Can you work these out from the model? Positions are in its coordinate system, mm. Round coordinates to 2 decimals unless told otherwise and drop trailing zeros. Loops run counter-clockwise (first coordinate to the right, second up) from the corner with the lowest first, then second, coordinate; pieces in that order, holes last.
(1) Thinking about a two-plate mould opening in Z: for faces 1 (the face through (0, 1, 30)), 2 (the face through (15.364, 0.72, -15.975)), 3 (the face through (1.936, 0.72, -13.536)), 4 (the face through (30, 1, 0)), which applies, released by +Z, released by -Z, zero draft, split by the parting line, or undercut?
(2) If I drill on line 1 along X through (y, z) = (0.4, 0) (3 decimals); line 2 along Z through (x, y) = (-14.96, 1.2) (3 decimals); line 3 along Z through (x, y) = (-27, 0.4), over which ranges is the centre line in solid material (lowest first)?
(3) I want a section at C-C on y = 0.5. Give the number of separate pieces and of enclosed holes in the cut face, plus the area to 3 significant figures.
(4) I want a section at B-B on z = 0. Write out the boundary of the cut face in (x, y) (3 decimals), plus the area to 3 significant figures.
(5) I want a section at A-A on z = 15. Write out the boundary of the cut face in (x, y) (3 decimals).
from build123d import *

# Parameters (mm, degrees)
SKETCH1_W           = 60
SKETCH1_H           = 60
SKETCH1_R           = 0.55
SKETCH1_R_2         = 1.465
SKETCH1_R_3         = 1.375
SKETCH1_R_4         = 1.055
BOSS_EXTRUDE1_DEPTH = 1.46


with BuildPart() as part:
    # Sketch1 → Boss-Extrude1 (new body)
    with BuildSketch(Plane(origin=(0, 0, 0), x_dir=(1, 0, 0), z_dir=(0, 1, 0))):
        Rectangle(SKETCH1_W, SKETCH1_H)
        with Locations(Location((-28.5, 28.5, 0), (0, 0, 270))):
            Circle(SKETCH1_R, mode=Mode.SUBTRACT)
        with Locations(Location((-27.968, 15, 0), (0, 0, 270))):
            Circle(SKETCH1_R_2, mode=Mode.SUBTRACT)
        with Locations(Location((-14.75, 0, 0), (0, 0, 270))):
            Circle(SKETCH1_R_3, mode=Mode.SUBTRACT)
        with Locations(Location((-14.960000108, 15, 0), (0, 0, 270))):
            Circle(SKETCH1_R_4, mode=Mode.SUBTRACT)
        with Locations(Location((-2, 15, 0), (0, 0, 270))):
            Circle(SKETCH1_R_2, mode=Mode.SUBTRACT)
        with Locations(Location((2, 15, 0), (0, 0, 90))):
            Circle(SKETCH1_R_2, mode=Mode.SUBTRACT)
        with Locations(Location((14.960000108, 15, 0), (0, 0, 90))):
            Circle(SKETCH1_R_4, mode=Mode.SUBTRACT)
        with Locations(Location((14.75, 0, 0), (0, 0, 90))):
            Circle(SKETCH1_R_3, mode=Mode.SUBTRACT)
        with Locations(Location((27.968, 15, 0), (0, 0, 90))):
            Circle(SKETCH1_R_2, mode=Mode.SUBTRACT)
        with Locations(Location((28.5, 28.5, 0), (0, 0, 90))):
            Circle(SKETCH1_R, mode=Mode.SUBTRACT)
        with Locations(Location((28.5, -28.5, 0), (0, 0, 270))):
            Circle(SKETCH1_R, mode=Mode.SUBTRACT)
        with Locations(Location((27.968, -15, 0), (0, 0, 270))):
            Circle(SKETCH1_R_2, mode=Mode.SUBTRACT)
        with Locations(Location((14.960000108, -15, 0), (0, 0, 270))):
            Circle(SKETCH1_R_4, mode=Mode.SUBTRACT)
        with Locations(Location((2, -15, 0), (0, 0, 270))):
            Circle(SKETCH1_R_2, mode=Mode.SUBTRACT)
        with Locations(Location((-2, -15, 0), (0, 0, 90))):
            Circle(SKETCH1_R_2, mode=Mode.SUBTRACT)
        with Locations(Location((-14.960000108, -15, 0), (0, 0, 90))):
            Circle(SKETCH1_R_4, mode=Mode.SUBTRACT)
        with Locations(Location((-27.968, -15, 0), (0, 0, 90))):
            Circle(SKETCH1_R_2, mode=Mode.SUBTRACT)
        with Locations(Location((-28.5, -28.5, 0), (0, 0, 90))):
            Circle(SKETCH1_R, mode=Mode.SUBTRACT)
    extrude(amount=BOSS_EXTRUDE1_DEPTH)


solid = part.part
Filled sheet:
1. face 1: released by +Z
1. face 2: undercut
1. face 3: undercut
1. face 4: zero draft
2. line 1: x = -30 to -16.125, -13.375 to 13.375, 16.125 to 30
2. line 2: z = -30 to -16.055, -13.945 to -1.359, 1.359 to 13.945, 16.055 to 30
2. line 3: z = -30 to -16.1, -13.9 to 13.9, 16.1 to 30
3. separate pieces: 1
3. enclosed holes: 18
3. area: 3,520 mm2
4. outline: (-30, 0) - (-16.125, 0) - (-16.125, 1.46) - (-30, 1.46) - close; (-13.375, 0) - (13.375, 0) - (13.375, 1.46) - (-13.375, 1.46) - close; (16.125, 0) - (30, 0) - (30, 1.46) - (16.125, 1.46) - close
4. area: 79.6 mm2
5. outline: (-30, 0) - (-29.433, 0) - (-29.433, 1.46) - (-30, 1.46) - close; (-26.503, 0) - (-16.015, 0) - (-16.015, 1.46) - (-26.503, 1.46) - close; (-13.905, 0) - (-3.465, 0) - (-3.465, 1.46) - (-13.905, 1.46) - close; (-0.535, 0) - (0.535, 0) - (0.535, 1.46) - (-0.535, 1.46) - close; (3.465, 0) - (13.905, 0) - (13.905, 1.46) - (3.465, 1.46) - close; (16.015, 0) - (26.503, 0) - (26.503, 1.46) - (16.015, 1.46) - close; (29.433, 0) - (30, 0) - (30, 1.46) - (29.433, 1.46) - close
